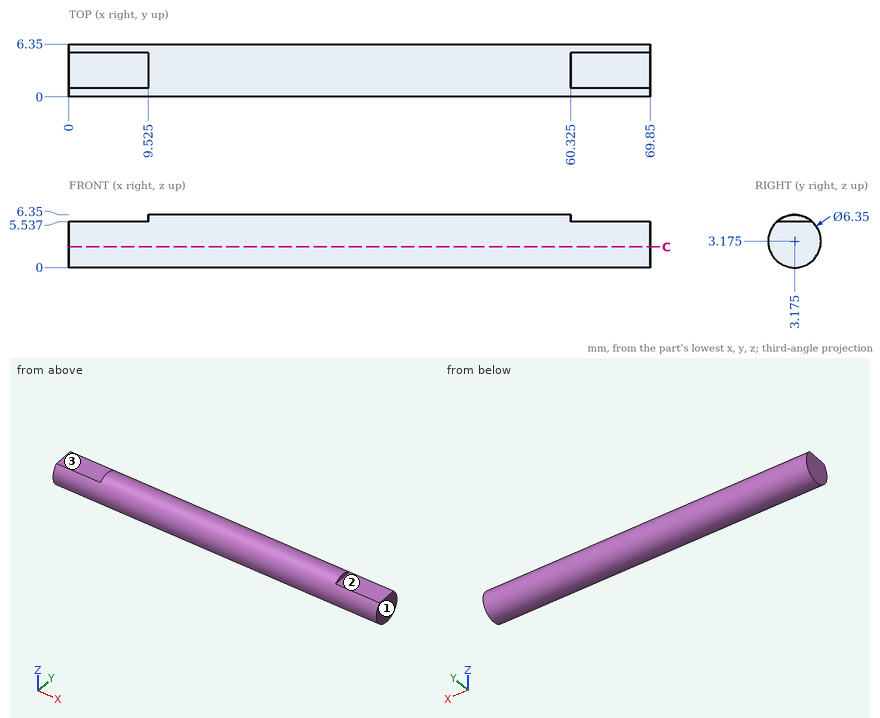
Study the drawing (mm; zero at the part's minimum x, y, z) and answer. A direction names the side the tool comes from. Coordinates: 2 decimals unless noted, no trailing zeros. Write each loop counter-clockwise with the first axis right and the second up, starting at its lowest first coordinate (ties: lowest second). Pieces come first, ordered by that corner, then holes.
Q1. A cutting plane is placed at C-C, the plane z = 2.5. Give the vertices of the cut face in (x, y), then the cut area to 3 significant figures.
Q2. Which of the six approach directions +Z, -Z, +X, -X, +Y, -Y give full straight-line access (tool end or side, diameter ignored) to the marked faces 1, 2 and 3?
Q3. Find the intervals of material crossed by line 1 (Z direction, x = 32, y = 3) (1 decimal); line 2 (Z direction, x = 53.5, y = 4.25), in increasing order.
Q4. This flat-tipped pin is pushed along its axis until it touches: pin 1 Ø1.3 at (x, y) = (66.5, 2) entering from +Z. Where does it stop, or does it pass through?
Findings below:
1. outline: (0, 0.07) - (69.85, 0.07) - (69.85, 6.28) - (0, 6.28) - close
1. area: 433 mm2
2. face 1: +Z, -Z, +X, +Y, -Y
2. face 2: +Z, +X, +Y, -Y
2. face 3: +Z, -X, +Y, -Y
3. line 1: z = 0 to 6.3
3. line 2: z = 0.19 to 6.16
4. pin 1: stops at z = 5.54
